Part model, mm, in its own coordinate system. Face numbers are marked on the shaded views. Coordinates: 2 decimals unless noted, no trailing zeros. Loops run counter-clockwise (first coordinate to the right, second up) from the corner with the lowest first, then second, coordinate; pieces in that order, holes last.
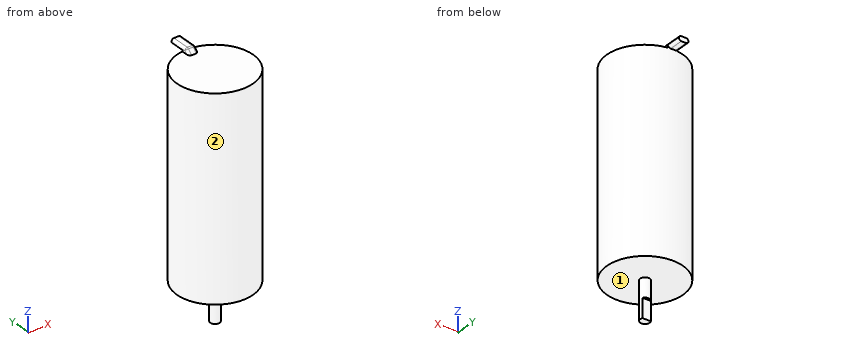
```python
from build123d import *

# Parameters (mm, degrees)
SKETCH1_R           = 8
BOSS_EXTRUDE1_DEPTH = 41.6
SKETCH2_W           = 2
SKETCH2_H           = 5
BOSS_EXTRUDE2_DEPTH = 1
CHAMFER1_SIZE       = 1
FILLET1_R           = 0.5
FILLET2_R           = 0.5
SKETCH3_R           = 1
BOSS_EXTRUDE3_DEPTH = 8
SKETCH4_W           = 2.782468735
SKETCH4_H           = 1.387929773
CUT_EXTRUDE1_DEPTH  = 4


# Some blends are built 0.0001 mm under size
with BuildPart() as part:
    # Sketch1 → Boss-Extrude1 (new body)
    with BuildSketch(Plane.XY):
        Circle(SKETCH1_R)
    extrude(amount=BOSS_EXTRUDE1_DEPTH)

    # Sketch2 → Boss-Extrude2 (add)
    with BuildSketch(Plane.XY.offset(41.6)):
        with Locations((0, 8.5)):
            Rectangle(SKETCH2_W, SKETCH2_H)
    extrude(amount=BOSS_EXTRUDE2_DEPTH)

    # Chamfer1
    chamfer1_edges = [part.edges().sort_by_distance(p)[0] for p in [
        (0, 6, 42.6),
    ]]
    chamfer(chamfer1_edges, length=CHAMFER1_SIZE - 0.0001)  # a hair under: the kernel refuses the full size

    # Fillet1
    fillet1_edges = [part.edges().sort_by_distance(p)[0] for p in [
        (1, 8.99995, 42.6),
        (0, 6.9999, 42.6),
        (1, 6.49995, 42.10005),
        (-1, 6.49995, 42.10005),
        (-1, 8.99995, 42.6),
    ]]
    fillet(fillet1_edges, radius=FILLET1_R)

    # Fillet2
    # the kernel refuses this fillet: 0.5 mm, written as the material it takes off along each edge
    with BuildSketch(Plane(origin=(-1, 6.687253933, 41.6), x_dir=(0, 0, 1), z_dir=(0, 1, 0))) as fillet2_piece_1_section:
        with BuildLine():
            CenterArc((FILLET2_R, FILLET2_R), FILLET2_R, 180, 90)
            Line((0, FILLET2_R), (-FILLET2_R * 0.02, FILLET2_R))
            Line((-FILLET2_R * 0.02, FILLET2_R), (-FILLET2_R * 0.02, -FILLET2_R * 0.02))
            Line((-FILLET2_R * 0.02, -FILLET2_R * 0.02), (FILLET2_R, -FILLET2_R * 0.02))
            Line((FILLET2_R, -FILLET2_R * 0.02), (FILLET2_R, 0))
        make_face()
    fillet2_piece_1 = extrude(amount=4.312746067, mode=Mode.PRIVATE)
    fillet2_piece_1 = split(fillet2_piece_1, bisect_by=Plane(origin=(-0.898582018, 9.474400051, 41.6), z_dir=(0, 0, 1)), keep=Keep.TOP, mode=Mode.PRIVATE)
    fillet2_piece_1 = fillet2_piece_1 - Plane(origin=(0, 0, 41.723690259), x_dir=(1, 0, 0), z_dir=(0, 0, -1)) * Cylinder(8, 11, mode=Mode.PRIVATE)
    add(fillet2_piece_1, mode=Mode.SUBTRACT)
    with BuildSketch(Plane(origin=(1, 11, 41.6), x_dir=(-1, 0, 0), z_dir=(0, -1, 0))) as fillet2_piece_2_section:
        with BuildLine():
            CenterArc((FILLET2_R, -FILLET2_R), FILLET2_R, 90, 90)
            Line((0, -FILLET2_R), (-FILLET2_R * 0.02, -FILLET2_R))
            Line((-FILLET2_R * 0.02, -FILLET2_R), (-FILLET2_R * 0.02, FILLET2_R * 0.02))
            Line((-FILLET2_R * 0.02, FILLET2_R * 0.02), (FILLET2_R, FILLET2_R * 0.02))
            Line((FILLET2_R, FILLET2_R * 0.02), (FILLET2_R, 0))
        make_face()
    fillet2_piece_2 = extrude(amount=4.312746067, mode=Mode.PRIVATE)
    fillet2_piece_2 = split(fillet2_piece_2, bisect_by=Plane(origin=(0.898581764, 9.474398488, 41.6), z_dir=(0, 0, 1)), keep=Keep.TOP, mode=Mode.PRIVATE)
    fillet2_piece_2 = fillet2_piece_2 - Plane(origin=(0, 0, 41.723690294), x_dir=(1, 0, 0), z_dir=(0, 0, -1)) * Cylinder(8, 11, mode=Mode.PRIVATE)
    add(fillet2_piece_2, mode=Mode.SUBTRACT)

    # Sketch3 → Boss-Extrude3 (add)
    with BuildSketch(Plane(origin=(0, 0, 0), x_dir=(-1, 0, 0), z_dir=(0, 0, -1))):
        with Locations(Location((0, 0, 0), (0, 0, 180))):
            Circle(SKETCH3_R)
    extrude(amount=BOSS_EXTRUDE3_DEPTH)

    # Sketch4 → Cut-Extrude1 (cut)
    with BuildSketch(Plane(origin=(0, 0, -8), x_dir=(-1, 0, 0), z_dir=(0, 0, -1))):
        with Locations((0.104073174, 1.193964887)):
            Rectangle(SKETCH4_W, SKETCH4_H)
    extrude(amount=-CUT_EXTRUDE1_DEPTH, mode=Mode.SUBTRACT)


solid = part.part
```
Q1. Saw through at B-B (y = 0). List the corners of the cut face in (x, z).
Q2. Mould opens along Y. For the marked faces 1 and 2 say: released by +Y, released by -Y, zero draft, split by the parting line, or undercut.
Q3. Probe line 1 (Z direction, x = 0.25, y = -1.5); line 2 (X direction, y = -4.75, z = 3); line 3 (X direction, y = -3.5, z = 3). List the from-to ranges inside material, lowest first.
Q4. Drop flat-ended pins along their axis: P1, Ø1.5, axis at x = -2, z = 24.5, coming from the +Y side; P2, Ø1.5, axis at x = -4.5, y = -3, coming from the -Z side; P3, Ø2, axis at y = 7, z = 24, coming from the -X side; P4, Ø8, axis at x = 0, y = -1.5, coming from the -Z side. Give the stop position or say it passes through.
Q5. Saw through at D-D (y = -6.25). List the corners of the cut face in (x, z), plus the area to 3 significant figures.
Q6. Saw through at C-C (z = 14.5). List the corners of the cut face in (x, y).
Checked values:
1. outline: (-8, 0) - (-1, 0) - (-1, -8) - (1, -8) - (1, 0) - (8, 0) - (8, 41.6) - (-8, 41.6) - close
2. face 1: zero draft
2. face 2: split by the parting line
3. line 1: z = 0 to 41.6
3. line 2: x = -6.44 to 6.44
3. line 3: x = -7.19 to 7.19
4. P1: stops at y = 7.9
4. P2: stops at z = 0
4. P3: stops at x = -5.29
4. P4: stops at z = -8
5. outline: (-4.99, 0) - (4.99, 0) - (4.99, 41.6) - (-4.99, 41.6) - close
5. area: 415 mm2
6. outline: circle Ø16 at (0, 0)
